Here's how the part is built. I have some questions about the finished solid (model axes, mm). Face numbers are marked on the shaded views. Give positions to 0.01 mm unless a question says otherwise; leave off trailing zeros. Order: outer loops, then holes, each group sorted by start corner. A loop starts at its lowest first (then second) coordinate and runs counter-clockwise, first axis right, second up. Notation, with made-up numbers: (77.25, 40) -> (132.25, 40) arc R15 ccw to (132.25, 56) -> close; hole circle Ø11 at (30, -17). An arc over 180 degrees is marked (long way). Write each question's results on one line, items separated by ' | '. Start each with the question number.
Q1. I need wall thicknesses on line 1 along Y through (x, z) = (0, -6); line 2 along X through (y, z) = (5, -5.25); line 3 along X through (y, z) = (-3, -8). Which ranges of each line are inside material? Lowest first, please. Write a range as [from, to].
Q2. I'm going to push flat-ended pins straight in: pin 1 (1.9 mm diameter, centred on x = -53, z = -5, fed in from -Y); pin 2 (1.9 mm diameter, centred on x = -52.5, z = -7, fed in from +Y); pin 3 (3 mm diameter, centred on x = 32, z = -6.5, fed in from +Y). Where does each tip first touch, or does it pass through?
Q3. Imagine slicing it at D-D, the plane y = 0. Please give me the cut outline in (x, z), then the cut area to 3 significant figures.
Q4. Imagine slicing it at B-B, the plane y = -33.5. Please give me the cut outline in (x, z).
Q5. Imagine slicing it at C-C, the plane x = 21.5. Please give me the cut outline in (y, z).
Q6. Thinking about a two-plate mould opening in X: for the marked faces 1, 2 and 3, which applies, pulls with the +X half, pulls with the -X half, needs draft (parallel to the pull), parting line crosses it, or undercut?
Q7. Imagine slicing it at A-A, the plane z = -4.25. Please give me the cut outline in (x, y), then the cut area to 3 significant figures.
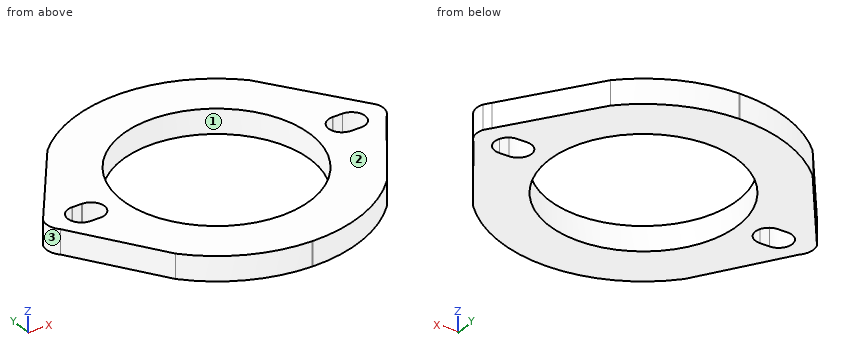
```python
from build123d import *

# Parameters (mm, degrees)
F0_R     = 38.5
F1_DEPTH = 10


# Not quite as in the source:
# - a feature names something its author has since deleted; it is built from what else it names


with BuildPart() as f1:
    # F0 (on Top) → F1 (new body)
    with BuildSketch(Plane.XY):
        with BuildLine():
            Line((-66.2866235273, -4.2965270375), (-42.9791214207, -39.2359080502))
            ThreePointArc((-42.9791214207, -39.2359080502), (-23.5911513271, -53.1988621842), (-0.226643991, -58.1945873009))
            ThreePointArc((-0.226643991, -58.1945873009), (0, -58.1950286418), (0.226643991, -58.1945873009))
            ThreePointArc((0.226643991, -58.1945873009), (23.5911513271, -53.1988621842), (42.9791214207, -39.2359080502))
            Line((42.9791214207, -39.2359080502), (66.2866235273, -4.2965270375))
            ThreePointArc((66.2866235273, -4.2965270375), (68.3602831702, -0.4175146073), (67.9024238921, 3.9570901325))
            Line((67.9024238921, 3.9570901325), (65.9713692122, 6.6390455982))
            Line((65.9713692122, 6.6390455982), (41.053212855, 41.2467583321))
            ThreePointArc((41.053212855, 41.2467583321), (22.3169041562, 53.7458570265), (0.2378206695, 58.1945426991))
            ThreePointArc((0.2378206695, 58.1945426991), (0, 58.1950286418), (-0.2378206695, 58.1945426991))
            ThreePointArc((-0.2378206695, 58.1945426991), (-22.3169041562, 53.7458570265), (-41.053212855, 41.2467583321))
            Line((-41.053212855, 41.2467583321), (-65.9713692122, 6.6390455982))
            Line((-65.9713692122, 6.6390455982), (-67.9024238921, 3.9570901325))
            ThreePointArc((-67.9024238921, 3.9570901325), (-68.3602831702, -0.4175146073), (-66.2866235273, -4.2965270375))
        make_face()
        with BuildLine():
            ThreePointArc((-55.0301875187, 5.4990596786), (-54.9860185236, 5.499237036), (-54.9418495285, 5.4990596786))
            Line((-54.9418495285, 5.4990596786), (-51.1476298855, 5.4990596786))
            ThreePointArc((-51.1476298855, 5.4990596786), (-51.013562259, 5.500693933), (-50.8794946326, 5.4990596786))
            ThreePointArc((-50.8794946326, 5.4990596786), (-45.5139634735, -0.065737976), (-51.0123484011, -5.499305933))
            Line((-51.0123484011, -5.499305933), (-54.9049202804, -5.5001650292))
            ThreePointArc((-54.9049202804, -5.5001650292), (-60.4856618743, -0.0633969362), (-55.0301875187, 5.4990596786))
        make_face(mode=Mode.SUBTRACT)
        Circle(F0_R, mode=Mode.SUBTRACT)
        with BuildLine():
            ThreePointArc((55.0301875187, 5.4990596786), (60.4856618743, -0.0633969362), (54.9049202804, -5.5001650292))
            Line((54.9049202804, -5.5001650292), (51.0123484011, -5.499305933))
            ThreePointArc((51.0123484011, -5.499305933), (45.5139634735, -0.065737976), (50.8794946326, 5.4990596786))
            ThreePointArc((50.8794946326, 5.4990596786), (51.013562259, 5.500693933), (51.1476298855, 5.4990596786))
            Line((51.1476298855, 5.4990596786), (54.9418495285, 5.4990596786))
            ThreePointArc((54.9418495285, 5.4990596786), (54.9860185236, 5.499237036), (55.0301875187, 5.4990596786))
        make_face(mode=Mode.SUBTRACT)
    extrude(amount=-F1_DEPTH)


solid = f1.part
```
Geometry check:
1) line 1: [-58.2, -38.5], [38.5, 58.2] | line 2: [-67.15, -57.28], [-48.72, -38.17], [38.17, 48.72], [57.28, 67.15] | line 3: [-67.33, -59.6], [-46.4, -38.38], [38.38, 46.4], [59.6, 67.33]
2) pin 1: y = -25.64 | pin 2: y = 26.67 | pin 3: y = 49.56
3) outline: (-68.43, -10) -> (-60.49, -10) -> (-60.49, 0) -> (-68.43, 0) -> close; (-45.51, -10) -> (-38.5, -10) -> (-38.5, 0) -> (-45.51, 0) -> close; (38.5, -10) -> (45.51, -10) -> (45.51, 0) -> (38.5, 0) -> close; (60.49, -10) -> (68.43, -10) -> (68.43, 0) -> (60.49, 0) -> close | area: 299 mm²
4) outline: (-46.81, -10) -> (-18.97, -10) -> (-18.97, 0) -> (-46.81, 0) -> close; (18.97, -10) -> (46.81, -10) -> (46.81, 0) -> (18.97, 0) -> close
5) outline: (-54.08, -10) -> (-31.94, -10) -> (-31.94, 0) -> (-54.08, 0) -> close; (31.94, -10) -> (54.08, -10) -> (54.08, 0) -> (31.94, 0) -> close
6) face 1: undercut | face 2: needs draft | face 3: pulls with the -X half
7) outline: (-67.9, 3.96) arc R7.5 ccw to (-66.29, -4.3) -> (-42.98, -39.24) arc R58.2 ccw to (42.98, -39.24) -> (66.29, -4.3) arc R7.5 ccw to (67.9, 3.96) -> (41.05, 41.25) arc R58.2 ccw to (0.24, 58.19) arc R58.2 ccw to (-0.24, 58.19) arc R58.2 ccw to (-41.05, 41.25) -> close; hole (-54.94, 5.5) arc R5.5 ccw (long way) to (-54.9, -5.5) -> (-51.01, -5.5) arc R5.5 ccw (long way) to (-51.15, 5.5) -> close; hole circle Ø77 at (0, 0); hole (51.01, -5.5) -> (54.9, -5.5) arc R5.5 ccw (long way) to (54.94, 5.5) -> (51.15, 5.5) arc R5.5 ccw (long way) to start | area: 6,160 mm²
